Model file for the job. Use its own axes, mm. Face numbers are marked on the shaded views. A direction names the side the tool comes from. Give positions to 0.01 mm unless a question says otherwise; leave off trailing zeros. Loops run counter-clockwise (first coordinate to the right, second up) from the corner with the lowest first, then second, coordinate; pieces in that order, holes last. Notation, with made-up numbers: M 85.5,78.25 L 94.5,78.25 A27 cw 94.5,106.25 Z; hole C 41,6 d7. An arc over 180 degrees is marked long. Use CSV: the item, a comma, the result in double quotes. Start each with the question number.
(1) Wall check: line 1 along Y through (x, z) = (171, 0) (3 decimals); line 2 along Z through (x, y) = (107.5, -1); line 3 along X through (y, z) = (-24, 8). Give the ranges that are in metal, low to high. Write a range as from..to.
(2) Tool access for the marked faces 1, 2 and 3: list every direction of +Z, -Z, +X, -X, +Y, -Y with a clear straight run to the whole face (end or side of a thin tool).
(3) Slice it at A-A on x = 132. List the corners of the cut face in (y, z), and give its area (3 significant figures).
(4) Flat gauge pins, fed straight in: P1, Ø4, axis at x = 104.5, z = -16.5, coming from the +Y side; P2, Ø8.5, axis at x = 3.5, z = -9.5, coming from the +Y side (3 decimals); P3, Ø8, axis at x = 44, z = -10.5, coming from the -Y side; P4, Ø11.5, axis at y = 21, z = 2.5, coming from the -X side. Where does each tip first touch, or does it go through?
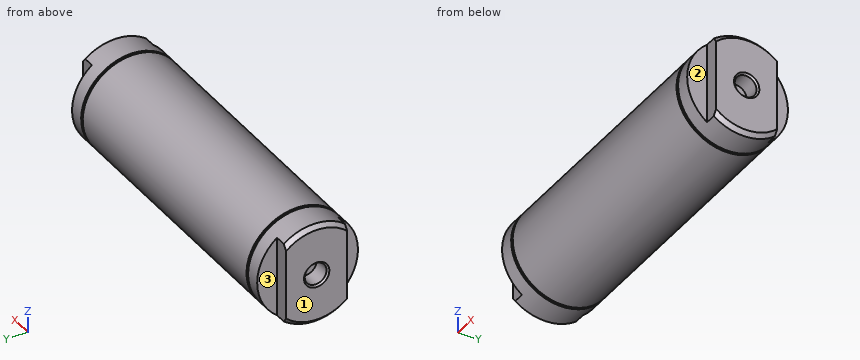
```python
from build123d import *

# Parameters (mm, degrees)
CUT_EXTRUDE1_START        = -7.9248
CUT_EXTRUDE1_DEPTH        = 7.9248
CUT_EXTRUDE2_START        = -7.9248
CUT_EXTRUDE2_DEPTH        = 7.9248
CUT_EXTRUDE3_DEPTH        = 7.9248
CUT_EXTRUDE4_DEPTH        = 7.9248
M10_CLEARANCE_HOLE1_D     = 11.35
M10_CLEARANCE_HOLE1_DEPTH = 9.50976
M10_CLEARANCE_HOLE2_D     = 11.35
M10_CLEARANCE_HOLE2_DEPTH = 9.50976
CHAMFER1_SIZE             = 2.094992
CHAMFER2_SIZE             = 0.9035


with BuildPart() as part:
    # Sketch1 → Revolve1 (revolve)
    with BuildSketch(Plane(origin=(0, 0, 0), x_dir=(-1, 0, 0), z_dir=(0, 0, -1)), mode=Mode.PRIVATE) as revolve1_sk:
        Polygon((-176.9872, 26.1874), (-176.9872, 0), (0, 0), (0, 26.1874), (-15.8496, 26.1874), (-15.8496, 25.632664), (-16.404336, 26.1874), (-16.800576, 25.79116), (-17.196816, 26.1874), (-159.790384, 26.1874), (-160.186624, 25.79116), (-160.582864, 26.1874), (-161.1376, 25.632664), (-161.1376, 26.1874), align=None)
    revolve(revolve1_sk.sketch.rotate(Axis((176.9872, 0, 0), (-1, 0, 0)), 270), axis=Axis((176.9872, 0, 0), (-1, 0, 0)))

    # Sketch2 → Cut-Extrude1 (cut)
    with BuildSketch(Plane.ZY.offset(CUT_EXTRUDE1_START)):
        with BuildLine():
            Line((-20.827008757, 15.875), (20.827008757, 15.875))
            ThreePointArc((20.827008757, 15.875), (0, 26.1874), (-20.827008757, 15.875))
        make_face()
    extrude(amount=CUT_EXTRUDE1_DEPTH, mode=Mode.SUBTRACT)

    # Sketch3 → Cut-Extrude2 (cut)
    with BuildSketch(Plane.ZY.offset(CUT_EXTRUDE2_START)):
        with BuildLine():
            Line((20.827008757, -15.875), (-20.827008757, -15.875))
            ThreePointArc((-20.827008757, -15.875), (0, -26.1874), (20.827008757, -15.875))
        make_face()
    extrude(amount=CUT_EXTRUDE2_DEPTH, mode=Mode.SUBTRACT)

    # Sketch4 → Cut-Extrude3 (cut)
    with BuildSketch(Plane(origin=(176.9872, 0, 0), x_dir=(0, 0, -1), z_dir=(1, 0, 0))):
        with BuildLine():
            Line((-20.827008757, 15.875), (20.827008757, 15.875))
            ThreePointArc((20.827008757, 15.875), (0, 26.1874), (-20.827008757, 15.875))
        make_face()
    extrude(amount=-CUT_EXTRUDE3_DEPTH, mode=Mode.SUBTRACT)

    # Sketch5 → Cut-Extrude4 (cut)
    with BuildSketch(Plane(origin=(176.9872, 0, 0), x_dir=(0, 0, -1), z_dir=(1, 0, 0))):
        with BuildLine():
            Line((20.827008757, -15.875), (-20.827008757, -15.875))
            ThreePointArc((-20.827008757, -15.875), (0, -26.1874), (20.827008757, -15.875))
        make_face()
    extrude(amount=-CUT_EXTRUDE4_DEPTH, mode=Mode.SUBTRACT)

    # M10 Clearance Hole1
    with Locations(Plane(origin=(176.9872, 0, 0), x_dir=(0, 0, -1), z_dir=(1, 0, 0))):
        with Locations((0, 0)):
            Hole(M10_CLEARANCE_HOLE1_D / 2, depth=M10_CLEARANCE_HOLE1_DEPTH)

    # M10 Clearance Hole2
    with Locations(Plane.ZY):
        with Locations((0, 0)):
            Hole(M10_CLEARANCE_HOLE2_D / 2, depth=M10_CLEARANCE_HOLE2_DEPTH)

    # Chamfer1
    chamfer1_edges = [part.edges().sort_by_distance(p)[0] for p in [
        (0, 0, -26.1874),
        (0, 8.377789375, 24.811137901),
        (176.9872, 0, -26.1874),
        (176.9872, 8.377789375, 24.811137901),
    ]]
    chamfer(chamfer1_edges, length=CHAMFER1_SIZE)

    # Chamfer2
    chamfer2_edges = [part.edges().sort_by_distance(p)[0] for p in [
        (176.9872, 0, -5.675),
        (0, 0, 5.675),
    ]]
    chamfer(chamfer2_edges, length=CHAMFER2_SIZE)


solid = part.part
```
Reply:
1,line 1,"y = -15.875..-5.675, 5.675..15.875"
1,line 2,"z = -26.17..26.17"
1,line 3,"x = 7.92..169.06"
2,face 1,"+Z, -Z, -X, +Y, -Y"
2,face 2,"+Z, -Z, +X, -Y"
2,face 3,"+Z, -Z, -X, +Y"
3,outline,"C 0,0 d52.37"
3,area,"2,150 mm^2"
4,P1,"stops at y = 21.81"
4,P2,"stops at y = 15.875"
4,P3,"stops at y = -25.37"
4,P4,"stops at x = 0"
